For this review, take the finished solid that the model builds, in its own axes (mm). A direction names the side the tool comes from. Give positions to 0.01 mm unless a question says otherwise; leave off trailing zeros. Loops run counter-clockwise (first coordinate to the right, second up) from the corner with the lowest first, then second, coordinate; pieces in that order, holes last. Notation, with made-up numbers: (-27.75, 34) -> (-11.75, 34) arc R31 cw to (-11.75, 68) -> close; hole circle Ø6 at (28.5, -25.75). An arc over 180 degrees is marked (long way). One line per question, with ' | ' between items. Start each with the question number.
(1) Draft analysis for pull direction X (two halves, no side actions). For faces 4 (the cylindrical face through (0, 12, 10)), 5 (the flat face through (12, 0, 0)), 6 (the cylindrical face through (17.084, 16.126, -3.794)), state which applies: +X half, -X half, draft (parallel to the pull), parting line (faces both ways), or undercut.
(2) Tool access review of faces 1 (the flat face through (3, 13, -11)), 2 (the flat face through (0, 7, 18)), 3 (the flat face through (8, 25, 8)): name each direction out of +Z, -Z, +X, -X, +Y, -Y from which nothing blocks a thin tool from reaching the whole face with its end or side.
(3) Wall thickness on probe 1 along X at (y, z) = (13, 0); probe 2 along Y at (x, z) = (17, 15.5); probe 3 along X at (y, z) = (5.25, 0): over which ranges is each line inside the solid? List them lowest first.
(4) Consider section D-D (z = -14). Write out the cut boundary in (x, y), and give its area (3 significant figures).
(5) Consider section A-A (z = 0). Write out the cut boundary in (x, y).
(6) Consider section B-B (x = 0). Write out the cut boundary in (y, z).
(7) Insertion check: P1, Ø1.8, axis at x = 0.5, y = 16, coming from the +Z side; P2, Ø1.5, axis at y = 16.5, z = -8, coming from the +X side; P3, Ø3, axis at y = 16, z = -10.5, coming from the -X side. Each pin has a flat end and moves straight along its axis. Give the tip position at first contact, or say it passes through.
(8) Consider section C-C (y = 6.25). Write out the cut boundary in (x, z).
from build123d import *

# Parameters (mm, degrees)
SKETCH_2_W          = 6
SKETCH_2_H          = 8.902136115
CUT_EXTRUDE_1_DEPTH = 46.639894829


with BuildPart() as part:
    # 草图1 → 旋转1 (revolve)
    with BuildSketch(Plane.XY, mode=Mode.PRIVATE) as revolve_1_sk:
        Polygon((10, 0), (27, 0), (27, 7), (17.5, 7), (17.5, 25), (10, 25), align=None)
    revolve(revolve_1_sk.sketch.rotate(Axis((0, 92.857139703, 0), (0, -1, 0)), 90), axis=Axis((0, 92.857139703, 0), (0, -1, 0)))

    # 草图2 → 切除-拉伸1 (cut, through all)
    with BuildSketch(Plane(origin=(0, 25, 0), x_dir=(1, 0, 0), z_dir=(0, 1, 0))):
        with Locations((0, 8.548931943)):
            Rectangle(SKETCH_2_W, SKETCH_2_H)
    extrude(amount=-CUT_EXTRUDE_1_DEPTH, mode=Mode.SUBTRACT)


solid = part.part
A:
1) face 4: undercut | face 5: draft | face 6: parting line
2) face 1: +Y, -Y | face 2: +Y | face 3: +Z, -Z, +X, -X, +Y
3) probe 1: x = -17.5 to -10, 10 to 17.5 | probe 2: y = 0 to 7 | probe 3: x = -27 to -10, 10 to 27
4) outline: (-23.09, 0) -> (23.09, 0) -> (23.09, 7) -> (10.5, 7) -> (10.5, 25) -> (-10.5, 25) -> (-10.5, 7) -> (-23.09, 7) -> close | area: 701 mm^2
5) outline: (-27, 0) -> (-10, 0) -> (-10, 25) -> (-17.5, 25) -> (-17.5, 7) -> (-27, 7) -> close; (10, 0) -> (27, 0) -> (27, 7) -> (17.5, 7) -> (17.5, 25) -> (10, 25) -> close
6) outline: (0, -27) -> (7, -27) -> (7, -17.5) -> (25, -17.5) -> (25, -13) -> (0, -13) -> close; (0, 10) -> (25, 10) -> (25, 17.5) -> (7, 17.5) -> (7, 27) -> (0, 27) -> close
7) P1: stops at z = 17.5 | P2: stops at x = 15.93 | P3: stops at x = -15.01
8) outline: circle Ø54 at (0, 0); hole (-3, -13) -> (3, -13) -> (3, -9.54) arc R10 ccw (long way) to (-3, -9.54) -> close
